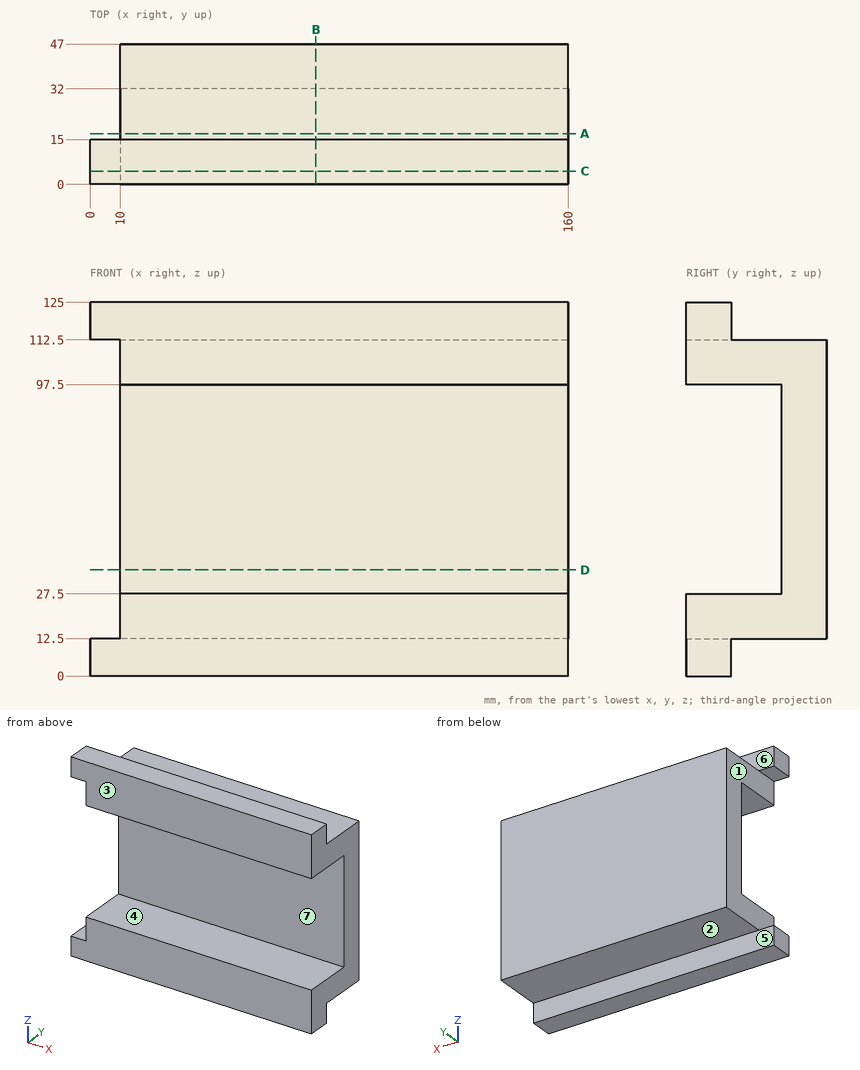
Geometry: see drawing. Coordinates: mm, zero at the bounding-box minimum. A direction names the side the tool comes from. Coordinates: 2 decimals unless noted, no trailing zeros. Order: outer loops, then holes, each group sorted by start corner. A loop starts at its lowest first (then second) coordinate and runs counter-clockwise, first axis right, second up. Notation, with made-up numbers: (30, -28.75) -> (89, -28.75) arc R26 ccw to (89, -13.75) -> close; hole circle Ø1 at (65, 8.25). An arc over 180 degrees is marked (long way). Write each question's results on one line, items separated by ' | '. Start each with the question number.
1) Mould query, pull axis Z, two halves, no side actions, for the marked faces 1, 2, 3 and 4. Classes: released by +Z, released by -Z, zero draft, split by the parting line, or undercut.
2) Cut plane D-D, the plane z = 35.5. Output: boundary loops of the cut face in (x, y), and give its area (3 significant figures).
3) Cut plane C-C, the plane y = 4.5. Output: boundary loops of the cut face in (x, z), and give its area (3 significant figures).
4) Material intervals for line 1 along Z through (x, y) = (104, 19.5); line 2 along Z through (x, y) = (34, 11); line 3 along X through (y, z) = (34, 19.5), sorted ascending.
5) Set-up query: the marked faces 5, 6 and 7. Return all of +Z, -Z, +X, -X, +Y, -Y with unobstructed straight access to the full face (end or side cutting, diameter ignored); none if empty.
6) Cut plane A-A, the plane y = 17. Output: boundary loops of the cut face in (x, z).
7) Cut plane B-B, the plane x = 75.5. Output: boundary loops of the cut face in (y, z), and give its area (4 significant figures).
8) First-contact query: pin 1 (8 mm diameter, centred on x = 17, y = 38, fed in from -Z); pin 2 (9.5 mm diameter, centred on x = 72.5, y = 24, fed in from +Z); pin 3 (12 mm diameter, centred on y = 34.5, z = 35, fed in from -X); pin 4 (10 mm diameter, centred on y = 17.5, z = 89.5, fed in from +X). Flat tips, straight axial feed; report the tip coordinate or a pass-through.
Checks:
1) face 1: undercut | face 2: released by -Z | face 3: zero draft | face 4: undercut
2) outline: (10, 32) -> (160, 32) -> (160, 47) -> (10, 47) -> close | area: 2,250 mm^2
3) outline: (0, 0) -> (160, 0) -> (160, 27.5) -> (10, 27.5) -> (10, 12.5) -> (0, 12.5) -> close; (0, 112.5) -> (10, 112.5) -> (10, 97.5) -> (160, 97.5) -> (160, 125) -> (0, 125) -> close | area: 8,500 mm^2
4) line 1: 12.5 to 27.5, 97.5 to 112.5 | line 2: 0 to 27.5, 97.5 to 125 | line 3: 10 to 160
5) face 5: -Z, +X, -X, +Y | face 6: +Z, +X, -X, +Y | face 7: +X, -X, -Y
6) outline: (10, 12.5) -> (160, 12.5) -> (160, 27.5) -> (10, 27.5) -> close; (10, 97.5) -> (160, 97.5) -> (160, 112.5) -> (10, 112.5) -> close
7) outline: (0, 0) -> (15, 0) -> (15, 12.5) -> (47, 12.5) -> (47, 112.5) -> (15, 112.5) -> (15, 125) -> (0, 125) -> (0, 97.5) -> (32, 97.5) -> (32, 27.5) -> (0, 27.5) -> close | area: 2,835 mm^2
8) pin 1: z = 12.5 | pin 2: z = 112.5 | pin 3: x = 10 | pin 4: through
